Could you check a few things on this model? Use its own coordinates, in mm. Face numbers are marked on the shaded views. Coordinates: 2 decimals unless noted, no trailing zeros. Loops run counter-clockwise (first coordinate to the right, second up) from the corner with the lowest first, then second, coordinate; pieces in that order, holes last.
1) Imagine slicing it at C-C on x = -16. Please give me the cut outline in (y, z).
2) Imagine slicing it at B-B on x = -11.75. Please give me the cut outline in (y, z), plus the area to 3 significant figures.
3) Imagine slicing it at A-A on z = 3.5. Please give me the cut outline in (x, y), plus the area to 3 significant figures.
4) Will this pin go through, and if not, where does the flat tip stop? P1, Ø1.5, axis at y = -20.5, z = 4.5, coming from the -X side.
5) Thinking about a two-plate mould opening in Y: for the marked faces 1, 2 and 3, which applies, released by +Y, released by -Y, zero draft, split by the parting line, or undercut?
6) Imagine slicing it at D-D on y = 6.5. Please give me the cut outline in (x, z).
7) If I drill on line 1 along Y through (x, z) = (-14.25, 3.75); line 2 along Z through (x, y) = (-10.5, -22); line 3 along Z through (x, y) = (-9, -25), over which ranges is the centre line in solid material (lowest first)?
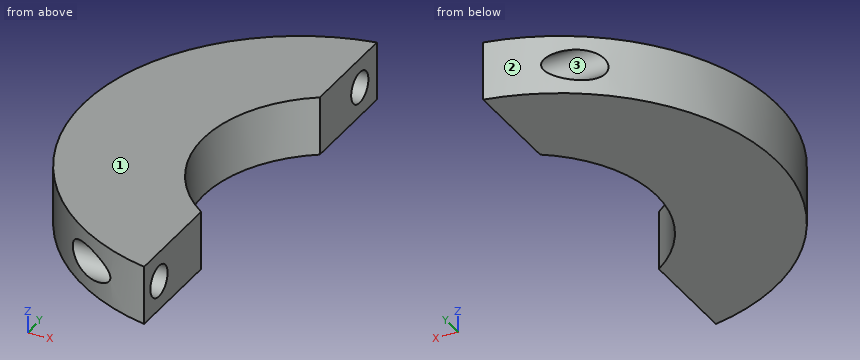
Autodesk Inventor part; units mm, degrees
ref_plane "YZ Plane" through (0, 0, 0) normal (1, 0, 0) x (0, 1, 0)
ref_plane "XZ Plane" through (0, 0, 0) normal (0, 1, 0) x (-1, 0, 0)
ref_plane "XY Plane" through (0, 0, 0) normal (0, 0, 1) x (1, 0, 0)
sketch "Sketch1" plane through (0, 0, 0) normal (0, 0, 1) x (1, 0, 0)
  arc A0 (0, 27.5) -> (0, -27.5) centre (0, 0) ccw
  arc A1 (-5, 13.7954) -> (-5, -13.7954) centre (4.5, 0) ccw
  line L0 (-5, -27.0416) -> (-5, -13.7954)
  arc A2 (-5, 27.0416) -> (-5, -27.0416) centre (0, 0) ccw
  line L1 (-5, 27.0416) -> (-5, 13.7954)
  point P0 (3.7885, 24.6247)
  point P1 (-3.7885, 24.6247)
  point P2 (-4.5, 0)
  point P3 (5, 27.5)
extrude "Extrusion1" add sketch "Sketch1" along normal blind 7.5
sketch "Sketch2" plane through (-5, -27.0416, 0) normal (1, 0, 0) x (0, 0, -1)
  line L0 (0, 6.9167) -> (7.5, 6.9167)
  line L1 (0, 0) -> (0, 6.9167)
  line L2 (0, 6.9167) -> (7.5, 6.9167)
  line L3 (7.5, 26.7893) -> (7.5, 0)
  line L4 (7.5, 6.9167) -> (7.5, 0)
  line L5 (7.5, 0) -> (0, 0)
  line L6 (7.5, 0) -> (0, 0)
  circle A0 centre (3.75, 3.4583) radius 1
  line L7 (0, 0) -> (3.0149, 2.7804)
  line L8 (4.4851, 4.1363) -> (7.5, 6.9167)
  line L9 (0, 6.9167) -> (3.0149, 4.1363)
  line L10 (4.4851, 2.7804) -> (7.5, 0)
  line L11 (0, 0) -> (0, 53.5786)
  line L12 (0, 53.5786) -> (0, 0)
  line L13 (0, 26.7893) -> (7.5, 26.7893)
  circle A1 centre (3.75, 50.1203) radius 1
  circle A2 centre (-3.75, 3.4583) radius 1
  circle A3 centre (-3.75, 50.1203) radius 1
  circle A4 centre (-3.75, 3.4583) radius 2
  circle A5 centre (-3.75, 50.1203) radius 2
  point P0 (0, 27.0416)
  point P1 (280.32, 51.414)
  dimension "d2" = 2
  dimension "d5" = 4
  dimension "d6" = 4
extrude "Extrusion2" cut sketch "Sketch2" against normal blind 25.4 contours A2 | A3
extrude "Extrusion3" cut sketch "Sketch2" against normal blind 18.575 contours A2 | A3 | A4 | A5
sketch "Sketch3" plane through (0, 0, 7.5) normal (0, 0, 1) x (1, 0, 0)
  line L0 (-5, 13.7954) -> (-5, 27.0416)
  arc A0 (-5, 27.0416) -> (-5, -27.0416) centre (0, 0) ccw
properties part number "Contrapeso5"
Filled in:
1. outline: (-22.37, 0) - (22.37, 0) - (22.37, 1.88) arc R2 cw to (22.37, 5.62) - (22.37, 7.5) - (-22.37, 7.5) - (-22.37, 5.34) arc R2 cw to (-22.37, 2.16) - close
2. outline: (-24.86, 0) - (-4.06, 0) - (-4.06, 7.5) - (-24.86, 7.5) - (-24.86, 5.29) arc R2 cw (long way) to (-24.86, 2.21) - close; (4.06, 0) - (24.86, 0) - (24.86, 2.85) arc R2 cw (long way) to (24.86, 4.65) - (24.86, 7.5) - (4.06, 7.5) - close
2. area: 289 mm2
3. outline: (-17.64, 21.09) arc R27.5 ccw to (-17.02, -21.6) - (-5, -21.6) - (-5, -13.8) arc R16.75 cw to (-5, 13.8) - (-5, 21.09) - close; (-11.32, 25.06) - (-5, 25.06) - (-5, 27.04) arc R27.5 ccw to start; (-10.13, -25.57) arc R27.5 ccw to (-5, -27.04) - (-5, -25.57) - close
3. area: 700 mm2
4. P1: stops at x = -19.14
5. face 1: zero draft
5. face 2: split by the parting line
5. face 3: undercut
6. outline: (-26.72, 0) - (-10.94, 0) - (-10.94, 7.5) - (-26.72, 7.5) - close
7. line 1: y = -21.58 to 21.08
7. line 2: z = 0 to 2.53, 4.97 to 7.5
7. line 3: z = 0 to 2.34, 5.16 to 7.5
